Geometry: see drawing. Coordinates: mm, zero at the bounding-box minimum. A direction names the side the tool comes from. Give positions to 0.01 mm unless a question says otherwise; leave off trailing zeros. Loops run counter-clockwise (first coordinate to the right, second up) from the corner with the lowest first, then second, coordinate; pieces in that order, holes last. Notation, with made-up numbers: (21.25, 69.25) -> (48.25, 69.25) arc R36 ccw to (48.25, 108.25) -> close; hole circle Ø2 at (39, 72.25). An arc over 180 degrees is marked (long way). One line per question, with ' | ' between items.
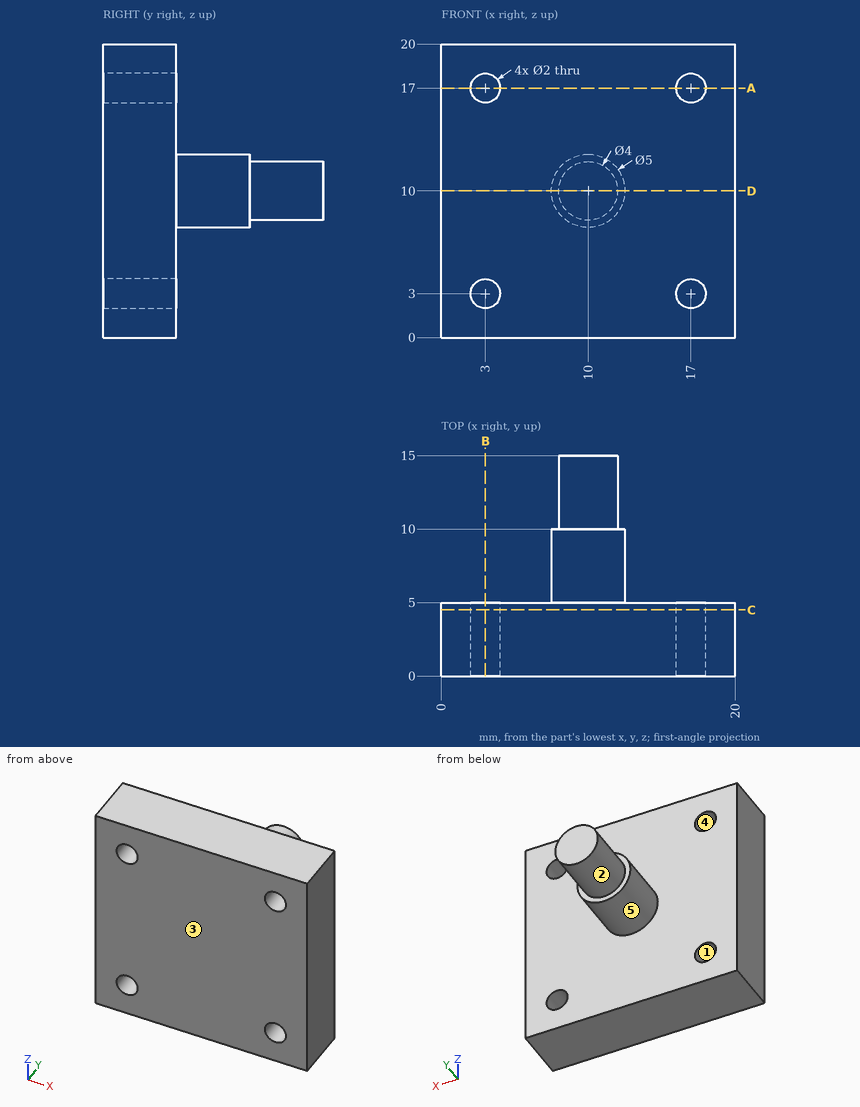
1. Pin query (flat end, axial travel): P1, Ø5, axis at x = 4, z = 14, coming from the +Y side; P2, Ø1.5, axis at x = 13, y = 8.5, coming from the +Z side; P3, Ø5, axis at y = 8, z = 14, coming from the -X side. Return the tip coordinate at first contact, or that it passes through.
Determined:
P1: stops at y = 5 | P2: stops at z = 11.09 | P3: stops at x = 8
2. Section query A-A (z = 17). Output: boundary loops of the cut face in (x, y), then the cut area to 3 significant figures.
Determined:
outline: (0, 0) -> (2, 0) -> (2, 5) -> (0, 5) -> close; (4, 0) -> (16, 0) -> (16, 5) -> (4, 5) -> close; (18, 0) -> (20, 0) -> (20, 5) -> (18, 5) -> close | area: 80.0 mm2
3. Pull-direction query (X, two-part tool) for the marked faces 1, 2 and 3; classes: pulls with the +X half, pulls with the -X half, needs draft (parallel to the pull), parting line crosses it, or undercut.
Determined:
face 1: undercut | face 2: parting line crosses it | face 3: needs draft
4. Reachability of the marked faces 4 and 5 from +Z, -Z, +X, -X, +Y, -Y: full face, straight path, thin tool, end or side. Return the list, or none.
Determined:
face 4: +Y, -Y | face 5: +Y
5. Section query B-B (x = 3). Output: boundary loops of the cut face in (y, z), then the cut area to 3 significant figures.
Determined:
outline: (0, 0) -> (5, 0) -> (5, 2) -> (0, 2) -> close; (0, 4) -> (5, 4) -> (5, 16) -> (0, 16) -> close; (0, 18) -> (5, 18) -> (5, 20) -> (0, 20) -> close | area: 80.0 mm2
6. Section query D-D (z = 10). Output: boundary loops of the cut face in (x, y), then the cut area to 3 significant figures.
Determined:
outline: (0, 0) -> (20, 0) -> (20, 5) -> (12.5, 5) -> (12.5, 10) -> (12, 10) -> (12, 15) -> (8, 15) -> (8, 10) -> (7.5, 10) -> (7.5, 5) -> (0, 5) -> close | area: 145 mm2
7. Section query C-C (y = 4.5). Output: boundary loops of the cut face in (x, z), then the cut area to 3 significant figures.
Determined:
outline: (0, 0) -> (20, 0) -> (20, 20) -> (0, 20) -> close; hole circle Ø2 at (3, 3); hole circle Ø2 at (3, 17); hole circle Ø2 at (17, 3); hole circle Ø2 at (17, 17) | area: 387 mm2
8. Ray query, line 1 along Y through (x, z) = (11.5, 5); line 2 along Z through (x, y) = (8.75, 12.5); line 3 along X through (y, z) = (5.25, 10.75). Return the intervals inside material, ascending. Write a range as from..to.
Determined:
line 1: y = 0..5 | line 2: z = 8.44..11.56 | line 3: x = 7.62..12.38
